Input: part model. Units: mm. Frame: model coordinates. Face numbers are marked on the shaded views. Coordinates: 2 decimals unless noted, no trailing zeros. Loops run counter-clockwise (first coordinate to the right, second up) from the corner with the lowest first, then second, coordinate; pieces in that order, holes last. Notation, with made-up numbers: (26.5, 8) -> (46.5, 8) arc R14 cw to (46.5, 20) -> close; hole circle Ø7 at (2.25, 79.5). An arc over 180 degrees is marked (long way). Put each result on its own line as item: value. Start each with the question number.
1) Material intervals for L1, parallel to X at y = 28.3, z = 10; L2, parallel to Z at x = -14, y = 29.3; L3, parallel to Z at x = -32.5, y = 4.2, sorted ascending.
2) Cut plane D-D (x = 0). Return the cut outline in (y, z), plus the area to 3 significant figures.
3) Cut plane B-B (y = 17). Return the cut outline in (x, z).
4) Cut plane C-C (x = -32.5). Return the cut outline in (y, z).
5) Pull-direction query (Z, two-part tool) for the marked faces 1 and 2; classes: pulls with the +Z half, pulls with the -Z half, needs draft (parallel to the pull), parting line crosses it, or undercut.
6) Contact query for flat-ended pins moving along their axis: P1, Ø16, axis at y = 24.5, z = 8.5, coming from the +X side; P2, Ø4, axis at x = -12.5, z = -24, coming from the +Y side; P3, Ø8, axis at x = 32.5, y = 19, coming from the +Z side. Output: stop coordinate, or through.
7) Cut plane A-A (z = 0). Return the cut outline in (x, y), plus the area to 3 significant figures.
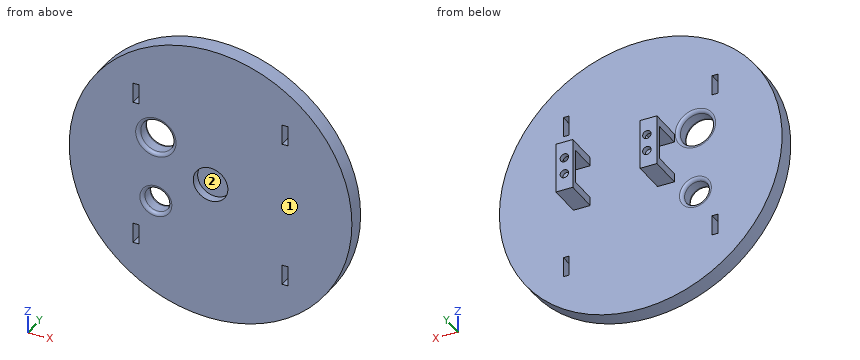
from build123d import *

# Parameters (mm, degrees)
SKETCH1_R               = 84
BASE_DEPTH              = 10
SKETCH3_W               = 10
SKETCH3_H               = 5
MOTOR_MOUNTS_BOTH_DEPTH = 20
SKETCH4_W               = 10
SKETCH4_H               = 20
SKETCH4_R               = 2.5
MOTOR_SCREW_HOLES_DEPTH = 3
SKETCH5_R               = 10.3
GEAR_HOLE_DEPTH         = 5.1
WIRE_HOLES_REACH        = 12
SKETCH6_R               = 7.5
SKETCH6_R_2             = 10
CUT_EXTRUDE1_REACH      = 12
FILLET2_R               = 2


with BuildPart() as part:
    # Sketch1 → base (new body)
    with BuildSketch(Plane(origin=(0, 0, 0), x_dir=(1, 0, 0), z_dir=(0, 1, 0))):
        Circle(SKETCH1_R)
    extrude(amount=BASE_DEPTH)

    # Sketch3 → motor mounts (both) (add)
    with BuildSketch(Plane(origin=(0, 10, 0), x_dir=(1, 0, 0), z_dir=(0, 1, 0))):
        with Locations((-15, 7.5)):
            Rectangle(SKETCH3_W, SKETCH3_H)
        with Locations((-15, -17.5)):
            Rectangle(SKETCH3_W, SKETCH3_H)
        with Locations((35, -17.5)):
            Rectangle(SKETCH3_W, SKETCH3_H)
        with Locations((35, 7.5)):
            Rectangle(SKETCH3_W, SKETCH3_H)
    extrude(amount=MOTOR_MOUNTS_BOTH_DEPTH)

    # Sketch4 → motor screw holes (add)
    with BuildSketch(Plane(origin=(0, 30, 0), x_dir=(1, 0, 0), z_dir=(0, 1, 0))):
        with Locations((-15, -5)):
            Rectangle(SKETCH4_W, SKETCH4_H)
        with Locations((-14, 0)):
            Circle(SKETCH4_R, mode=Mode.SUBTRACT)
        with Locations((-14, -10)):
            Circle(SKETCH4_R, mode=Mode.SUBTRACT)
        with Locations((35, -5)):
            Rectangle(SKETCH4_W, SKETCH4_H)
        with Locations((35, 0)):
            Circle(SKETCH4_R, mode=Mode.SUBTRACT)
        with Locations((35, -10)):
            Circle(SKETCH4_R, mode=Mode.SUBTRACT)
    extrude(amount=-MOTOR_SCREW_HOLES_DEPTH)

    # Sketch5 → gear hole (cut)
    with BuildSketch(Plane.XZ):
        Circle(SKETCH5_R)
    extrude(amount=-GEAR_HOLE_DEPTH, mode=Mode.SUBTRACT)

    # Sketch6 → wire holes (cut, up to next)
    with BuildSketch(Plane(origin=(0, 10, 0), x_dir=(1, 0, 0), z_dir=(0, 1, 0)), mode=Mode.PRIVATE) as wire_holes_sk1:
        with Locations((-32.5, 20)):
            Circle(SKETCH6_R)
    wire_holes_tool1 = extrude(wire_holes_sk1.sketch, amount=-WIRE_HOLES_REACH, mode=Mode.PRIVATE) & part.part
    add(wire_holes_tool1.solids().sort_by_distance((-32.5, 10, -20))[0], mode=Mode.SUBTRACT)
    # Sketch6 → wire holes (cut, up to next)
    with BuildSketch(Plane(origin=(0, 10, 0), x_dir=(1, 0, 0), z_dir=(0, 1, 0)), mode=Mode.PRIVATE) as wire_holes_sk2:
        with Locations((-32.5, -20)):
            Circle(SKETCH6_R_2)
    wire_holes_tool2 = extrude(wire_holes_sk2.sketch, amount=-WIRE_HOLES_REACH, mode=Mode.PRIVATE) & part.part
    add(wire_holes_tool2.solids().sort_by_distance((-32.5, 10, 20))[0], mode=Mode.SUBTRACT)

    # Sketch7 → Cut-Extrude1 (cut, up to next)
    with BuildSketch(Plane(origin=(0, 10, 0), x_dir=(1, 0, 0), z_dir=(0, 1, 0)), mode=Mode.PRIVATE) as cut_extrude1_sk1:
        Polygon((-42.5, 38), (-42.5, 47.5), (-42.5, 50), (-46, 50), (-46, 38), align=None)
    cut_extrude1_tool1 = extrude(cut_extrude1_sk1.sketch, amount=-CUT_EXTRUDE1_REACH, mode=Mode.PRIVATE) & part.part
    add(cut_extrude1_tool1.solids().sort_by_distance((-44.25, 10, -44))[0], mode=Mode.SUBTRACT)
    # Sketch7 → Cut-Extrude1 (cut, up to next)
    with BuildSketch(Plane(origin=(0, 10, 0), x_dir=(1, 0, 0), z_dir=(0, 1, 0)), mode=Mode.PRIVATE) as cut_extrude1_sk2:
        Polygon((42.5, 50), (42.5, 47.5), (42.5, 38), (46, 38), (46, 50), align=None)
    cut_extrude1_tool2 = extrude(cut_extrude1_sk2.sketch, amount=-CUT_EXTRUDE1_REACH, mode=Mode.PRIVATE) & part.part
    add(cut_extrude1_tool2.solids().sort_by_distance((44.25, 10, -44))[0], mode=Mode.SUBTRACT)
    # Sketch7 → Cut-Extrude1 (cut, up to next)
    with BuildSketch(Plane(origin=(0, 10, 0), x_dir=(1, 0, 0), z_dir=(0, 1, 0)), mode=Mode.PRIVATE) as cut_extrude1_sk3:
        Polygon((46, -38), (42.5, -38), (42.5, -47.5), (42.5, -50), (46, -50), align=None)
    cut_extrude1_tool3 = extrude(cut_extrude1_sk3.sketch, amount=-CUT_EXTRUDE1_REACH, mode=Mode.PRIVATE) & part.part
    add(cut_extrude1_tool3.solids().sort_by_distance((44.25, 10, 44))[0], mode=Mode.SUBTRACT)
    # Sketch7 → Cut-Extrude1 (cut, up to next)
    with BuildSketch(Plane(origin=(0, 10, 0), x_dir=(1, 0, 0), z_dir=(0, 1, 0)), mode=Mode.PRIVATE) as cut_extrude1_sk4:
        Polygon((-42.5, -47.5), (-42.5, -38), (-46, -38), (-46, -50), (-42.5, -50), align=None)
    cut_extrude1_tool4 = extrude(cut_extrude1_sk4.sketch, amount=-CUT_EXTRUDE1_REACH, mode=Mode.PRIVATE) & part.part
    add(cut_extrude1_tool4.solids().sort_by_distance((-44.25, 10, 44))[0], mode=Mode.SUBTRACT)

    # Fillet2
    fillet2_edges = [part.edges().sort_by_distance(p)[0] for p in [
        (-40, 10, -20),
        (-40, 0, -20),
        (-42.5, 10, 20),
        (-42.5, 0, 20),
    ]]
    fillet(fillet2_edges, radius=FILLET2_R)


solid = part.part
Results found:
1. L1: x = -20 to -16.5, -11.5 to -10, 30 to 32.5, 37.5 to 40
1. L2: z = -10 to -2.5, 2.5 to 7.5, 12.5 to 20
1. L3: z = -77.46 to -27.5, -12.5 to 10, 30 to 77.46
2. outline: (0, -84) -> (10, -84) -> (10, 84) -> (0, 84) -> (0, 10.3) -> (5.1, 10.3) -> (5.1, -10.3) -> (0, -10.3) -> close
2. area: 1,570 mm2
3. outline: (-20, -10) -> (-10, -10) -> (-10, -5) -> (-20, -5) -> close; (-20, 15) -> (-10, 15) -> (-10, 20) -> (-20, 20) -> close; (30, -10) -> (40, -10) -> (40, -5) -> (30, -5) -> close; (30, 15) -> (40, 15) -> (40, 20) -> (30, 20) -> close
4. outline: (0, -77.46) -> (10, -77.46) -> (10, -29.5) arc R2 ccw to (8, -27.5) -> (2, -27.5) arc R2 ccw to (0, -29.5) -> close; (0, -10.5) arc R2 ccw to (2, -12.5) -> (8, -12.5) arc R2 ccw to (10, -10.5) -> (10, 8) arc R2 ccw to (8, 10) -> (2, 10) arc R2 ccw to (0, 8) -> close; (0, 32) arc R2 ccw to (2, 30) -> (8, 30) arc R2 ccw to (10, 32) -> (10, 77.46) -> (0, 77.46) -> close
5. face 1: needs draft
5. face 2: undercut
6. P1: stops at x = 40
6. P2: stops at y = 10
6. P3: stops at z = 20
7. outline: (-84, 0) -> (-10.3, 0) -> (-10.3, 5.1) -> (10.3, 5.1) -> (10.3, 0) -> (84, 0) -> (84, 10) -> (-84, 10) -> close; (-20, 27) -> (-16.5, 27) -> (-16.5, 30) -> (-20, 30) -> close; (-11.5, 27) -> (-10, 27) -> (-10, 30) -> (-11.5, 30) -> close; (30, 27) -> (32.5, 27) -> (32.5, 30) -> (30, 30) -> close; (37.5, 27) -> (40, 27) -> (40, 30) -> (37.5, 30) -> close
7. area: 1,600 mm2
